The model under review builds one solid part; all positions refer to its coordinate system, in mm. A direction names the side the tool comes from. Round coordinates to 2 decimals unless told otherwise and drop trailing zeros. Order: outer loops, then holes, each group sorted by start corner. A loop starts at its lowest first (then second) coordinate and runs counter-clockwise, first axis right, second up.
```python
from build123d import *

# Parameters (mm, degrees)
BOSS_EXTRUDE2_START = -23.18385
BOSS_EXTRUDE2_DEPTH = 23.18385


with BuildPart() as part:
    # Sketch1 → Revolve1 (revolve)
    with BuildSketch(Plane.XY, mode=Mode.PRIVATE) as revolve1_sk:
        Polygon((-0.9906, 0), (-2.9845, 0), (-2.9845, 28.64485), (-0.9906, 33.47085), (-0.3429, 33.47085), (-0.3429, 9.31545), (-0.9906, 8.193600692), align=None)
    revolve(revolve1_sk.sketch.rotate(Axis((0, 0, 0), (0, 1, 0)), 270), axis=Axis((0, 0, 0), (0, 1, 0)))

    # Sketch2 → Boss-Extrude2 (add)
    with BuildSketch(Plane.XZ.offset(BOSS_EXTRUDE2_START)):
        with BuildLine():
            Line((2.9845, 2.9845), (-1e-09, 2.9845))
            ThreePointArc((-1e-09, 2.9845), (2.110360188, 2.110360189), (2.9845, 0))
            Line((2.9845, 0), (2.9845, 2.9845))
        make_face()
        with BuildLine():
            Line((-1e-09, 2.9845), (-2.9845, 2.9845))
            Line((-2.9845, 2.9845), (-2.9845, 5e-09))
            ThreePointArc((-2.9845, 5e-09), (-2.110360187, 2.11036019), (-1e-09, 2.9845))
        make_face()
        with BuildLine():
            Line((2.9845, -2.9845), (2.9845, 0))
            ThreePointArc((2.9845, 0), (2.110360188, -2.110360189), (-2e-09, -2.9845))
            Line((-2e-09, -2.9845), (2.9845, -2.9845))
        make_face()
        with BuildLine():
            ThreePointArc((-2e-09, -2.9845), (-2.110360191, -2.110360186), (-2.9845, 5e-09))
            Line((-2.9845, 5e-09), (-2.9845, -2.9845))
            Line((-2.9845, -2.9845), (-2e-09, -2.9845))
        make_face()
    extrude(amount=BOSS_EXTRUDE2_DEPTH)


solid = part.part
```
(1) For faces 5 (the cylindrical face through (1.14, 25.95, -2.76)), 6 (the flat face through (2.4, 23.184, -2.4)), 7 (the flat face through (2.3, 23.184, 2.4)), list the 3-axis set-ups (+Z, -Z, +X, -X, +Y, -Y) from which the entire face can be reached by the end or side of a thin tool; tool diameter is ignored.
Data:
face 5: +Y
face 6: -Z, +X, +Y
face 7: +Z, +X, +Y
(2) Consider section A-A (y = 6). Write out the cut boundary in (x, z), and give its area (3 significant figures).
Data:
outline: (-2.98, -2.98) - (2.98, -2.98) - (2.98, 2.98) - (-2.98, 2.98) - close; hole circle Ø1.98 at (0, 0)
area: 32.5 mm2
(3) To check wall thickness, follow probe 1 along X at (y, z) = (27.5, 0); probe 2 along X at (y, z) = (5, 0); probe 3 along Z at (x, y) = (-0.55, 8.5). State the ranges of each line that lie inside material, in increasing order.
Data:
probe 1: x = -2.98 to -0.34, 0.34 to 2.98
probe 2: x = -2.98 to -0.99, 0.99 to 2.98
probe 3: z = -2.98 to -0.6, 0.6 to 2.98
(4) Draft analysis for pull direction X (two halves, no side actions). For faces 1 (the cylindrical face through (-0.982, 4.039, 0.129)), 2 (the conical face through (0.515, 8.996, 0.114)), 3 (the flat face through (-1, 0, 1)), 4 (the flat face through (-2.984, 12, 0)), state which applies: pulls with the +X half, pulls with the -X half, needs draft (parallel to the pull), parting line crosses it, or undercut.
Data:
face 1: undercut
face 2: undercut
face 3: needs draft
face 4: pulls with the -X half
(5) Insertion check: pin 1 (2.5 mm diameter, centred on x = 1.5, z = -2, fed in from +Y). The pin has a flat end and moves straight along its axis. Give the tip position at first contact, or say it passes through.
Data:
pin 1: stops at y = 32.84
